Design review of the part built by this model. Coordinates are the model's own, in mm. A direction names the side the tool comes from. Coordinates: 2 decimals unless noted, no trailing zeros. Loops run counter-clockwise (first coordinate to the right, second up) from the corner with the lowest first, then second, coordinate; pieces in that order, holes last. Notation, with made-up numbers: M -16.75,75.5 L 3.25,75.5 A8 cw 3.25,83.5 Z; hole C 52,52 d6. An arc over 180 degrees is marked long. Write item = value, one per line. Start each with the question number.
from build123d import *


with BuildPart() as f1:
    # F0 (on Front) → F1 (revolve)
    with BuildSketch(Plane.XZ):
        with BuildLine():
            Line((-57.507594, 8), (-62.5, 8))
            Line((-62.5, 8), (-62.5, 0))
            Line((-62.5, 0), (-20.108948, 0))
            Line((-20.108948, 0), (19.891052, 0))
            Line((19.891052, 0), (62.5, 0))
            Line((62.5, 0), (62.5, 8))
            Line((62.5, 8), (57.492453, 8))
            Line((57.492453, 8), (57.492453, 5))
            Line((57.492453, 5), (52.492453, 5))
            Line((52.492453, 5), (52.492453, 8))
            Line((52.492453, 8), (19.891052, 8))
            Line((19.891052, 8), (19.891052, 96))
            ThreePointArc((19.891052, 96), (18.426586, 99.535534), (14.891052, 101))
            Line((14.891052, 101), (-15.108948, 101))
            ThreePointArc((-15.108948, 101), (-18.644481, 99.535534), (-20.108948, 96))
            Line((-20.108948, 96), (-20.108948, 8))
            Line((-20.108948, 8), (-52.507594, 8))
            Line((-52.507594, 8), (-52.507594, 5))
            Line((-52.507594, 5), (-57.507594, 5))
            Line((-57.507594, 5), (-57.507594, 8))
        make_face()
    revolve(axis=Axis((-6.764503, 0, 0), (1, 0, 0)))


solid = f1.part
Q1. To check wall thickness, follow line 1 (Y direction, x = -15, z = -2); line 2 (X direction, y = -84, z = -1); line 3 (Y direction, x = 40, z = 0). State the ranges of each line that lie inside material, in increasing order. Write a range as from..to.
Q2. Mouldability with a two-part tool opening along X and no side actions: class faces 5 (the face through (62.5, 0, 0)), 6 (the face through (59.96, 7.81, -1.73)), 7 (the face through (-57.508, 5.2, 0.1)), 8 (the face through (-20.109, -1, 20)) as released by +X, released by -X, zero draft, split by the parting line, or undercut.
Q3. For faces 1 (the face through (-60.04, 7.81, -1.73)), 2 (the face through (52.492, 5.2, 0.1)), 3 (the face through (-62.5, 0, 0)), 4 (the face through (35.96, 7.81, -1.73)), list the 3-axis set-ups (+Z, -Z, +X, -X, +Y, -Y) from which the entire face can be reached by the end or side of a thin tool; tool diameter is ignored.
Q4. Add section C-C on x = 27.5. State the section outline as (y, z) points, plus the area to 3 significant figures.
Q5. Clearance check with flat-ended pins moving along their axes: P1, Ø12, axis at y = -25, z = -52, coming from the +X side; P2, Ø5, axis at y = 32.5, z = -3, coming from the -X side; P3, Ø3, axis at x = 10.5, z = -79.5, coming from the +Y side; P4, Ø1.5, axis at x = 49.5, y = 10, coming from the -Z side. State where each tip first meets the part, or that it passes through.
Values follow:
q1.line_1 = -100.98..100.98
q1.line_2 = -20.11..19.89
q1.line_3 = -8..8
q2.face_5 = released by +X
q2.face_6 = zero draft
q2.face_7 = undercut
q2.face_8 = released by -X
q3.face_1 = -X
q3.face_2 = none
q3.face_3 = +Z, -Z, -X, +Y, -Y
q3.face_4 = +X
q4.outline = C 0,0 d16
q4.area = 201 mm2
q5.P1 = 19.89
q5.P2 = -20.11
q5.P3 = 64.16
q5.P4 = through
